```python
from build123d import *

# Parameters (mm, degrees)
SKETCH1_W               = 125
SKETCH1_H               = 125
BOSS_EXTRUDE1_DEPTH     = 0.15
CUT_EXTRUDE1_DEPTH      = 89.388474927
MIRROR2_COPY_1_DEPTH    = 89.388474927
SKETCH4_W               = 3
SKETCH4_H               = 5.4
BOSS_EXTRUDE2_DEPTH     = 0.01
LPATTERN1_COUNT         = 2
LPATTERN1_PITCH         = 38.5
LPATTERN1_COL_COUNT     = 2
LPATTERN1_COL_PITCH     = 38.5
MIRROR3_COPY_1_SKETCH_W = 3
MIRROR3_COPY_1_SKETCH_H = 5.4
MIRROR3_COPY_1_DEPTH    = 0.01
MIRROR3_COPY_2_SKETCH_W = 3
MIRROR3_COPY_2_SKETCH_H = 5.4
MIRROR3_COPY_2_DEPTH    = 0.01


with BuildPart() as part:
    # Sketch1 → Boss-Extrude1 (new body)
    with BuildSketch(Plane.XY):
        Rectangle(SKETCH1_W, SKETCH1_H)
    extrude(amount=BOSS_EXTRUDE1_DEPTH)

    # Sketch2 → Cut-Extrude1 (cut, through all)
    with BuildSketch(Plane.XY.offset(0.15)):
        Polygon((-62.5, 50.63708499), (-50.63708499, 62.5), (-62.5, 62.5), align=None)
    cut_extrude1 = extrude(amount=-CUT_EXTRUDE1_DEPTH, mode=Mode.SUBTRACT)

    # Mirror1: Cut-Extrude1 across plane
    add(cut_extrude1.mirror(Plane.ZX), mode=Mode.SUBTRACT)

    # Mirror2: Cut-Extrude1 across plane
    add(cut_extrude1.mirror(Plane(origin=(0, 0, 0), x_dir=(0, 0, 1), z_dir=(1, 0, 0))), mode=Mode.SUBTRACT)

    # Mirror2 copy 1 sketch → Mirror2 copy 1 (cut, through all)
    with BuildSketch(Plane(origin=(0, 0, 0.15), x_dir=(-1, 0, 0), z_dir=(0, 0, 1))):
        Polygon((-62.5, 50.63708499), (-50.63708499, 62.5), (-62.5, 62.5), align=None)
    extrude(amount=-MIRROR2_COPY_1_DEPTH, mode=Mode.SUBTRACT)

    # Sketch4 → Boss-Extrude2 (add)
    with BuildSketch(Plane(origin=(0, 0, 0), x_dir=(-1, 0, 0), z_dir=(0, 0, -1))):
        with Locations((0, 59.8)):
            Rectangle(SKETCH4_W, SKETCH4_H)
    boss_extrude2 = extrude(amount=BOSS_EXTRUDE2_DEPTH)

    # LPattern1: Boss-Extrude2 ×2
    with Locations(*[(-i * LPATTERN1_PITCH, 0, 0) for i in range(1, LPATTERN1_COUNT)]):
        add(boss_extrude2)

    # LPattern1 col: Boss-Extrude2 ×2
    with Locations(*[(i * LPATTERN1_COL_PITCH, 0, 0) for i in range(1, LPATTERN1_COL_COUNT)]):
        add(boss_extrude2)

    # Mirror3: Boss-Extrude2 across plane
    add(boss_extrude2.mirror(Plane.ZX))

    # Mirror3 copy 1 sketch → Mirror3 copy 1 (add)
    with BuildSketch(Plane(origin=(-38.5, 0, 0), x_dir=(-1, 0, 0), z_dir=(0, 0, -1))):
        with Locations((0, -59.8)):
            Rectangle(MIRROR3_COPY_1_SKETCH_W, MIRROR3_COPY_1_SKETCH_H)
    extrude(amount=MIRROR3_COPY_1_DEPTH)

    # Mirror3 copy 2 sketch → Mirror3 copy 2 (add)
    with BuildSketch(Plane(origin=(38.5, 0, 0), x_dir=(-1, 0, 0), z_dir=(0, 0, -1))):
        with Locations((0, -59.8)):
            Rectangle(MIRROR3_COPY_2_SKETCH_W, MIRROR3_COPY_2_SKETCH_H)
    extrude(amount=MIRROR3_COPY_2_DEPTH)


solid = part.part
```
Build history of the part. All positions in model axes, mm. Coordinates: 2 decimals unless noted, no trailing zeros. Order: outer loops, then holes, each group sorted by start corner. A loop starts at its lowest first (then second) coordinate and runs counter-clockwise, first axis right, second up. Notation, with made-up numbers: M 43.25,85 L 57.25,85 A13 cw 57.25,89 Z; hole C -36,3 d2. An arc over 180 degrees is marked long. One line per question, with ' | ' between items. Start each with the question number.
1. Wall check: line 1 along Z through (x, y) = (43, -37.5); line 2 along Y through (x, z) = (-52.5, 0.1); line 3 along Y through (x, z) = (52, 0.1). Give the ranges that are in metal, low to high. Write a range as [from, to].
2. Cut at B-B (x = -28.5). Write the cut outline in (y, z), plus the area to 4 significant figures.
3. Flat gauge pin, fed straight in: P1, Ø6, axis at x = 44.5, y = 29, coming from the -Z side. Where does the tip first touch, or does it go through?
4. Cut at A-A (z = 0.1). Write the cut outline in (x, y), plus the area to 3 significant figures.
The answers:
1) line 1: z = [0, 0.15] | line 2: y = [-60.64, 60.64] | line 3: y = [-61.14, 61.14]
2) outline: M -62.5,0 L 62.5,0 L 62.5,0.15 L -62.5,0.15 Z | area: 18.75 mm2
3) P1: stops at z = 0
4) outline: M -62.5,-50.64 L -50.64,-62.5 L 50.64,-62.5 L 62.5,-50.64 L 62.5,50.64 L 50.64,62.5 L -50.64,62.5 L -62.5,50.64 Z | area: 15,300 mm2
